Autodesk Inventor part; units mm, degrees
ref_plane "YZ Plane" through (0, 0, 0) normal (1, 0, 0) x (0, 1, 0)
ref_plane "XZ Plane" through (0, 0, 0) normal (0, 1, 0) x (-1, 0, 0)
ref_plane "XY Plane" through (0, 0, 0) normal (0, 0, 1) x (1, 0, 0)
sketch "Sketch1" plane through (0, 0, 0) normal (1, 0, 0) x (0, 1, 0)
  circle A0 centre (0, 0) radius 45
  dimension "d0" = 90
extrude "Extrusion1" add sketch "Sketch1" along normal mid plane 12
sketch "Sketch2" plane through (6, 0, 0) normal (1, 0, 0) x (0, 0, -1)
  circle A0 centre (0, 0) radius 30
  circle A1 centre (0, 0) radius 22.5
  dimension "d3" = 60
  dimension "d4" = 45
extrude "Extrusion2" add sketch "Sketch2" along normal blind 3
sketch "Sketch3" plane through (-6, 0, 0) normal (-1, 0, 0) x (0, 0, 1)
  circle A0 centre (0, 0) radius 19
  dimension "d7" = 38
extrude "Extrusion3" add sketch "Sketch3" along normal blind 3
sketch "Sketch4" plane through (6, 0, 0) normal (1, 0, 0) x (0, 0, -1)
  circle A0 centre (0, 0) radius 8
  circle A1 centre (0, 37.5) radius 4
  circle A2 centre (-37.5, 0) radius 4
  circle A3 centre (0, -37.5) radius 4
  circle A4 centre (37.5, 0) radius 4
  dimension "d10" = 16
  dimension "d11" = 8
  dimension "d12" = 37.5
  dimension "d15" = 360
  dimension "d17" = 75
  dimension "d18" = 37.5
extrude "Extrusion4" cut sketch "Sketch4" against normal through all
Design review of the part built by this model. Coordinates are the model's own, in mm. A direction names the side the tool comes from. Give positions to 0.01 mm unless a question says otherwise; leave off trailing zeros. Order: outer loops, then holes, each group sorted by start corner. A loop starts at its lowest first (then second) coordinate and runs counter-clockwise, first axis right, second up. Notation, with made-up numbers: (19, 53) - (30, 53) arc R20 ccw to (30, 90) - close; hole circle Ø6 at (88.25, 76). An arc over 180 degrees is marked (long way). Use CSV: the item, a comma, the result in double quotes. Start each with the question number.
Q1. Take a section at B-B (x = -4.5). State the section outline as (y, z) points.
Q2. For line 1 (Y direction, x = 3.25, z = -35); line 2 (X direction, y = 4, z = -27.5); line 3 (X direction, y = -22, z = -27.5), list the stretches that pass through material, from the lowest coordinate up.
Q3. Take a section at C-C (z = -35.5). State the section outline as (x, y) points.
Q4. Take a section at A-A (y = 0). State the section outline as (x, z) points.
Q5. Machinability: for faces 1 (the face through (6, 0, -10)), 2 (the face through (-7.479, 16.856, 8.767)), 3 (the face through (0.1, -2.4, -34.3)), which of the approach directions +Z, -Z, +X, -X, +Y, -Y give a long, thin tool a straight path to every point of the face, cutting with its end or side? Answer none if there is none.
Q6. Draft analysis for pull direction Z (two halves, no side actions). For faces 4 (the face through (-6, -0.6, -19.4)), 5 (the face through (-0.084, 20.765, 39.923)), 6 (the face through (0.084, -33.534, 0.521)), state which applies: pulls with the +Z half, pulls with the -Z half, needs draft (parallel to the pull), parting line crosses it, or undercut.
Q7. For P1, Ø5, axis at y = 0, z = -37.5, coming from the -X side; P2, Ø10, axis at x = -2.5, y = 31, coming from the +Z side; P3, Ø8, axis at x = 1, y = 9.5, coming from the +Z side; P4, Ø2, axis at x = -3.5, z = -32.5, coming from the +Y side, all flat-tipped, find the tip position at first contact; note any pin that passes through.
Q8. Take a section at D-D (y = 37.5). State the section outline as (x, z) points.
Calculated:
1,outline,"circle Ø90 at (0, 0); hole circle Ø8 at (-37.5, 0); hole circle Ø16 at (0, 0); hole circle Ø8 at (0, -37.5); hole circle Ø8 at (0, 37.5); hole circle Ø8 at (37.5, 0)"
2,line 1,"y = -28.28 to -3.12, 3.12 to 28.28"
2,line 2,"x = -6 to 9"
2,line 3,"x = -6 to 6"
3,outline,"(-6, -27.65) - (6, -27.65) - (6, -3.46) - (-6, -3.46) - close; (-6, 3.46) - (6, 3.46) - (6, 27.65) - (-6, 27.65) - close"
4,outline,"(-9, -19) - (-6, -19) - (-6, -33.5) - (6, -33.5) - (6, -30) - (9, -30) - (9, -22.5) - (6, -22.5) - (6, -8) - (-9, -8) - close; (-9, 8) - (6, 8) - (6, 22.5) - (9, 22.5) - (9, 30) - (6, 30) - (6, 33.5) - (-6, 33.5) - (-6, 19) - (-9, 19) - close; (-6, -45) - (6, -45) - (6, -41.5) - (-6, -41.5) - close; (-6, 41.5) - (6, 41.5) - (6, 45) - (-6, 45) - close"
5,face 1,"+X"
5,face 2,"-X"
5,face 3,"+X, -X"
6,face 4,"needs draft"
6,face 5,"parting line crosses it"
6,face 6,"undercut"
7,P1,"passes through"
7,P2,"stops at z = 36.73"
7,P3,"stops at z = 44.66"
7,P4,"stops at y = 32.14"
8,outline,"(-6, -24.87) - (6, -24.87) - (6, -4) - (-6, -4) - close; (-6, 4) - (6, 4) - (6, 24.87) - (-6, 24.87) - close"
